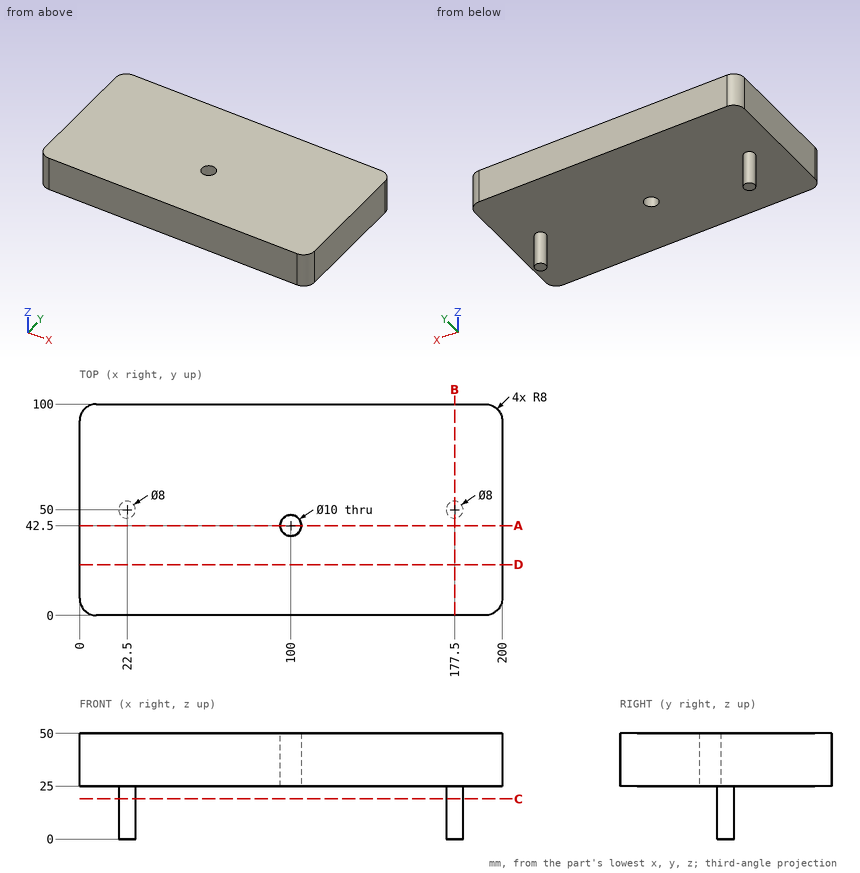
Can you work these out from the drawing? Everything is in mm from the part's minimum corner. Give positions to 0.01 mm unless a question says otherwise; leave off trailing zeros. Order: outer loops, then holes, each group sorted by start corner. A loop starts at its lowest first (then second) coordinate and runs counter-clockwise, first axis right, second up. Notation, with made-up numbers: M 9,86.25 L 18,86.25 A18 cw 18,93.25 Z; hole C -7.75,15.25 d8. An arc over 180 degrees is marked long. One line per question, with ' | ' between items.
1. I want a section at B-B (x = 177.5). List the corners of the cut face in (y, z) for me.
Results:
outline: M 0,25 L 46,25 L 46,0 L 54,0 L 54,25 L 100,25 L 100,50 L 0,50 Z
2. I'm going to push flat-ended pins straight in: pin 1 (3 mm diameter, centred on x = 142, y = 84.5, fed in from -Z); pin 2 (8 mm diameter, centred on x = 100, y = 42.5, fed in from -Z). Where does each tip first touch, or does it pass through?
Results:
pin 1: z = 25 | pin 2: through
3. I want a section at D-D (y = 24). List the corners of the cut face in (x, z) for me.
Results:
outline: M 0,25 L 200,25 L 200,50 L 0,50 Z
4. I want a section at A-A (y = 42.5). List the corners of the cut face in (x, z) for me, and give its area (3 significant figures).
Results:
outline: M 0,25 L 95,25 L 95,50 L 0,50 Z; M 105,25 L 200,25 L 200,50 L 105,50 Z | area: 4,750 mm²
5. I want a section at C-C (z = 19). List the corners of the cut face in (x, y) for me.
Results:
outline: C 22.5,50 d8; C 177.5,50 d8
6. If I drill on line 1 (Y direction, x = 100, z = 35); line 2 (X direction, y = 42.5, z = 37.75); line 3 (Z direction, x = 171, y = 60.5), over which ranges is the centre line in solid material (lowest first)?
Results:
line 1: 0 to 37.5, 47.5 to 100 | line 2: 0 to 95, 105 to 200 | line 3: 25 to 50
